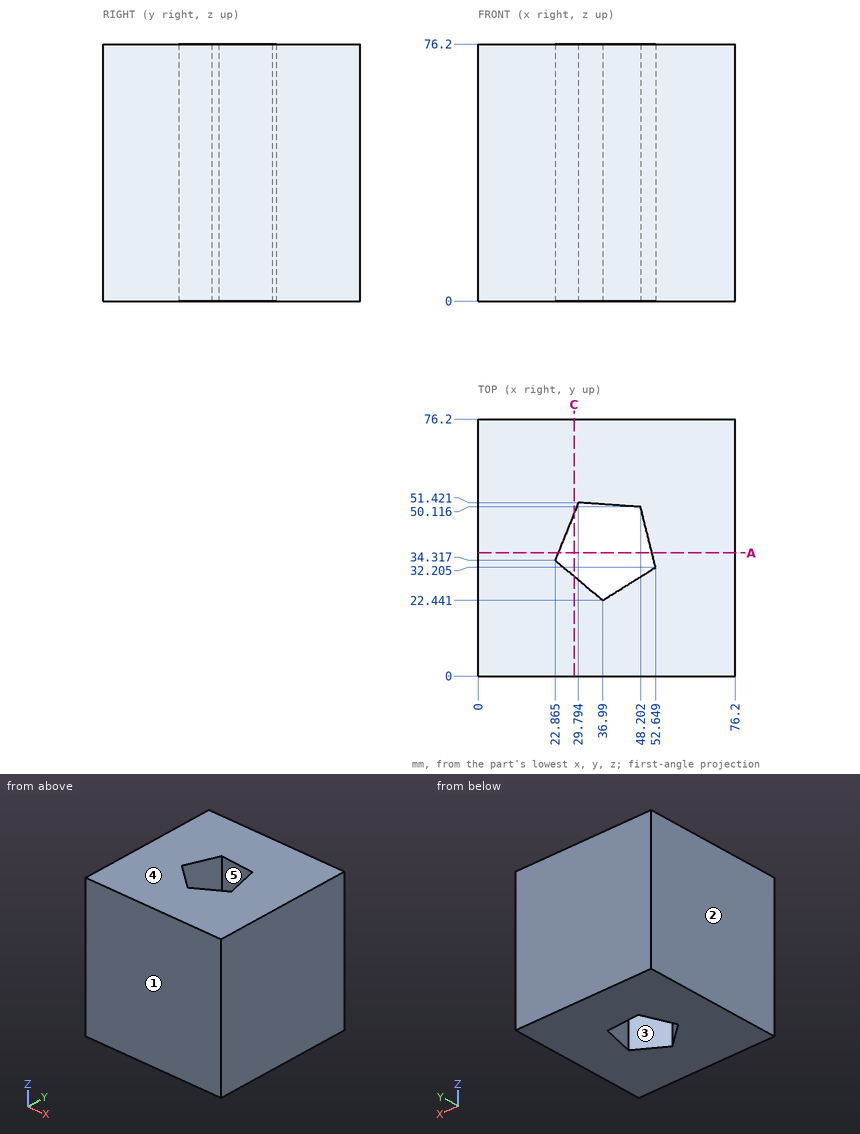
Geometry check sheet. Reference: drawing and pictorial views, mm from the part's lowest x, y, z. A direction names the side the tool comes from. Round coordinates to 2 decimals unless told otherwise and drop trailing zeros. Loops run counter-clockwise (first coordinate to the right, second up) from the corner with the lowest first, then second, coordinate; pieces in that order, holes last.
1. Set-up check for the marked faces 4 and 5: record each of +Z, -Z, +X, -X, +Y, -Y from which the full face is reachable in a straight line by a thin tool's end or side.
2. Sectioned sample at A-A on y = 36.5. Record the boundary of the cut face in (x, z).
3. Mould release check, pull along Y, two halves, no side actions. Record for the marked faces 1, 2 and 3: released by +Y, released by -Y, zero draft, split by the parting line, or undercut.
4. Gauge pin test, flat end, axial feed: pin 1 Ø10 at (x, y) = (33.5, 41) entering from -Z. Record the tip position at first contact, or that the pin passes through.
5. Sectioned sample at C-C on x = 28.5. Record the boundary of the cut face in (y, z), and give its area (3 significant figures).
6. Scan lines: probe 1 along Y at (x, z) = (40, 32); probe 2 along Y at (x, z) = (25.5, 66.5) (1 decimal); probe 3 along X at (y, z) = (48, 52). Record each from-to range of solid material in increasing order.
Recorded:
1. face 4: +Z, +X, -X, +Y, -Y
1. face 5: +Z, -Z
2. outline: (0, 0) - (23.75, 0) - (23.75, 76.2) - (0, 76.2) - close; (51.58, 0) - (76.2, 0) - (76.2, 76.2) - (51.58, 76.2) - close
3. face 1: released by -Y
3. face 2: zero draft
3. face 3: undercut
4. pin 1: passes through
5. outline: (0, 0) - (29.58, 0) - (29.58, 76.2) - (0, 76.2) - close; (48.23, 0) - (76.2, 0) - (76.2, 76.2) - (48.23, 76.2) - close
5. area: 4,390 mm2
6. probe 1: y = 0 to 24.32, 50.7 to 76.2
6. probe 2: y = 0 to 32.1, 40.8 to 76.2
6. probe 3: x = 0 to 28.41, 48.73 to 76.2
